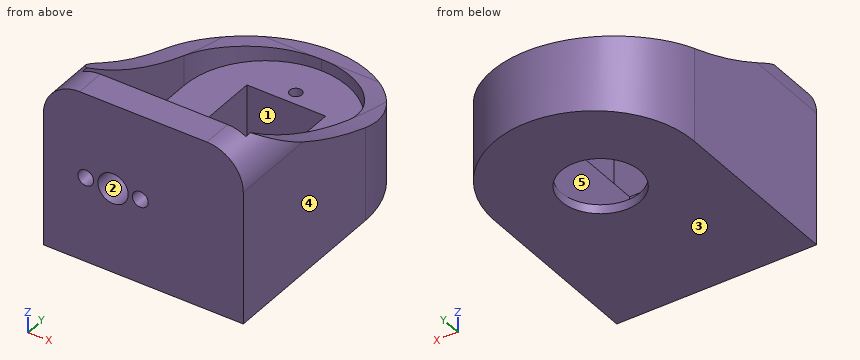
```python
from build123d import *

# Parameters (mm, degrees)
SKETCH1_W           = 33
SKETCH1_H           = 28
BOSS_EXTRUDE1_DEPTH = 46
SKETCH2_W           = 17.5
SKETCH2_H           = 41
CUT_EXTRUDE1_DEPTH  = 46
BOSS_EXTRUDE2_DEPTH = 3
BOSS_EXTRUDE3_DEPTH = 27
FILLET1_START       = -3.5
FILLET1_DEPTH       = 5.015993094
FILLET1_START_2     = -13.5
FILLET1_2_DEPTH     = 27
FILLET2_R           = 16.5
FILLET3_R           = 6
SKETCH5_W           = 13
SKETCH5_H           = 23
CUT_EXTRUDE4_DEPTH  = 9
SKETCH6_R           = 6.5
CUT_EXTRUDE5_DEPTH  = 9
SKETCH7_R           = 1
CUT_EXTRUDE6_DEPTH  = 8
SKETCH8_R           = 1.3
SKETCH8_R_2         = 2.5
CUT_EXTRUDE7_DEPTH  = 47.360004936


with BuildPart() as part:
    # Sketch1 → Boss-Extrude1 (new body)
    with BuildSketch(Plane(origin=(0, 0, 0), x_dir=(1, 0, 0), z_dir=(0, 1, 0))):
        Rectangle(SKETCH1_W, SKETCH1_H)
    extrude(amount=BOSS_EXTRUDE1_DEPTH)

    # Sketch2 → Cut-Extrude1 (cut)
    with BuildSketch(Plane(origin=(16.5, 0, 0), x_dir=(0, 0, -1), z_dir=(1, 0, 0))):
        with Locations((-5.25, 25.5)):
            Rectangle(SKETCH2_W, SKETCH2_H)
    extrude(amount=-CUT_EXTRUDE1_DEPTH, mode=Mode.SUBTRACT)

    # Sketch3 → Boss-Extrude2 (add)
    with BuildSketch(Plane(origin=(16.5, 0, 0), x_dir=(0, 0, -1), z_dir=(1, 0, 0))):
        with BuildLine():
            Line((3.5, 46), (2, 46))
            add(Edge.make_bspline(
                [(-14, 5), (-0.68227026, 23.158489921), (2, 46)],
                knots=[0, 0, 0, 1, 1, 1], degree=2))
            Line((-14, 5), (3.5, 5))
            Line((3.5, 5), (3.5, 46))
        make_face()
    boss_extrude2 = extrude(amount=-BOSS_EXTRUDE2_DEPTH)

    # Mirror1: Boss-Extrude2 across plane
    add(boss_extrude2.mirror(Plane(origin=(0, 0, 0), x_dir=(0, 0, 1), z_dir=(1, 0, 0))))

    # Sketch4 → Boss-Extrude3 (add)
    with BuildSketch(Plane.ZY.offset(-13.5)):
        with BuildLine():
            Line((-3.5, 46), (-3.5, 43))
            Line((-3.5, 43), (-1.598813094, 43))
            add(Edge.make_bspline(
                [(-1.598813094, 43), (-1.82265352, 44.489763885), (-2.000000005, 46.000000046)],
                knots=[0.933881948, 0.933881948, 0.933881948, 1, 1, 1], degree=2))
            Line((-2.000000005, 46.000000046), (-3.5, 46))
        make_face()
    extrude(amount=BOSS_EXTRUDE3_DEPTH)

    # Fillet1: read off the stored shape, not the designer's step
    # Fillet1 outline → Fillet1 (add)
    with BuildSketch(Plane.XY.offset(FILLET1_START)):
        with BuildLine():
            ThreePointArc((-13.5, 29.5), (-9.545941546, 39.045941546), (0, 43))
            Line((0, 43), (-13.5, 43))
            Line((-13.5, 43), (-13.5, 29.5))
        make_face()
        with BuildLine():
            ThreePointArc((0, 43), (9.545941546, 39.045941546), (13.5, 29.5))
            Line((13.5, 29.5), (13.5, 43))
            Line((13.5, 43), (0, 43))
        make_face()
    extrude(amount=FILLET1_DEPTH)

    # Fillet1 2 outline → Fillet1 2 (cut)
    with BuildSketch(Plane.YZ.offset(FILLET1_START_2)):
        with BuildLine():
            add(Edge.make_bspline(
                [(43, -1.598813094), (36.02565956, -0.550902514), (29.499999971, 1.515993003)],
                knots=[0.066118051, 0.066118051, 0.066118051, 0.375650194, 0.375650194, 0.375650194], degree=2))
            Line((43, -1.598813094), (43, 1.515993094))
            Line((43, 1.515993094), (29.499999971, 1.515993003))
        make_face()
    extrude(amount=FILLET1_2_DEPTH, mode=Mode.SUBTRACT)

    # Fillet2
    # the kernel refuses this fillet: 16.5 mm, written as the material it takes off along each edge
    with BuildSketch(Plane(origin=(16.5, 46, -55.25), x_dir=(0, -1, 0), z_dir=(0, 0, 1)), Plane(origin=(-16.5, 46, 39.25), x_dir=(0, -1, 0), z_dir=(0, 0, -1))) as fillet2_piece_1:
        with BuildLine():
            CenterArc((FILLET2_R, -FILLET2_R), FILLET2_R, 90, 90)
            Line((0, -FILLET2_R), (0, 0))
            Line((0, 0), (FILLET2_R, 0))
        make_face()
    extrude(amount=94.5, mode=Mode.SUBTRACT)

    # Fillet3
    # the kernel refuses this fillet: 6 mm, written as the material it takes off along each edge
    with BuildSketch(Plane(origin=(-16.5, -15, 14), x_dir=(1, 0, 0), z_dir=(0, 1, 0)), Plane(origin=(16.5, -15, 14), x_dir=(0, 0, -1), z_dir=(0, 1, 0))) as fillet3_piece_1:
        with BuildLine():
            CenterArc((FILLET3_R, FILLET3_R), FILLET3_R, 180, 90)
            Line((0, FILLET3_R), (0, 0))
            Line((0, 0), (FILLET3_R, 0))
        make_face()
    extrude(amount=35, mode=Mode.SUBTRACT)

    # Sketch5 → Cut-Extrude4 (cut)
    with BuildSketch(Plane.XY.offset(-3.5)):
        with Locations((0, 23)):
            Rectangle(SKETCH5_W, SKETCH5_H)
    extrude(amount=-CUT_EXTRUDE4_DEPTH, mode=Mode.SUBTRACT)

    # Sketch6 → Cut-Extrude5 (cut)
    with BuildSketch(Plane.XY.offset(-12.5)):
        with Locations((0, 28)):
            Circle(SKETCH6_R)
    extrude(amount=-CUT_EXTRUDE5_DEPTH, mode=Mode.SUBTRACT)

    # Sketch7 → Cut-Extrude6 (cut)
    with BuildSketch(Plane.XY.offset(-3.5)):
        with Locations((0, 36.8)):
            Circle(SKETCH7_R)
        with Locations((0, 9.2)):
            Circle(SKETCH7_R)
    extrude(amount=-CUT_EXTRUDE6_DEPTH, mode=Mode.SUBTRACT)

    # Sketch8 → Cut-Extrude7 (cut, through all)
    with BuildSketch(Plane(origin=(0, 5, 0), x_dir=(1, 0, 0), z_dir=(0, 1, 0))):
        with Locations(Location((-0.5, 0, 0), (0, 0, 270))):
            Circle(SKETCH8_R)
        with Locations(Location((-5, 0, 0), (0, 0, 270))):
            Circle(SKETCH8_R_2)
        with Locations(Location((-9.5, 0, 0), (0, 0, 270))):
            Circle(SKETCH8_R)
    extrude(amount=-CUT_EXTRUDE7_DEPTH, mode=Mode.SUBTRACT)


solid = part.part
```
Work out the finished part from the listing and answer in its coordinate system (mm). Face numbers are marked on the shaded views. A direction names the side the tool comes from. Coordinates: 2 decimals unless noted, no trailing zeros. Use CSV: the item, a comma, the result in double quotes.
1) Consider line 1 (X direction, y = 20, z = 1.25); line 2 (X direction, y = 2, z = 0); line 3 (X direction, y = 28, z = -13.45). Determine where each line is inside the solid, lowest interval first. Write a range as [from, to].
Worked out:
line 1,"x = [-16.5, -13.5], [13.5, 16.5]"
line 2,"x = [-16.5, -10.8], [-8.2, -7.5], [-2.5, -1.8], [0.8, 16.5]"
line 3,"x = [-16.5, -6.5], [6.5, 16.5]"
2) For the marked faces 4 and 5, determine the directions among +Z, -Z, +X, -X, +Y, -Y from which every point of the face is accessible in a straight line to the end or side of a thin tool.
Worked out:
face 4,"+Z, -Z, +X, +Y, -Y"
face 5,"+Z"
3) Section A-A on x = -5 is taken. Count the separate pieces of the cut face and the enclosed holes in it, plus the area to 3 significant figures.
Worked out:
separate pieces,"3"
enclosed holes,"0"
area,"324 mm^2"
4) Determine the mould class of the marked faces 1, 2 and 3 for opening direction Z: released by +Z, released by -Z, zero draft, split by the parting line, or undercut.
Worked out:
face 1,"zero draft"
face 2,"undercut"
face 3,"released by -Z"
5) Flat-ended cylindrical pins translate along their axes: pin 1 Ø5 at (x, z) = (-9, -9.5) entering from -Y; pin 2 Ø0.6 at (x, y) = (0, 36.5) entering from +Z; pin 3 Ø5 at (x, y) = (-4.5, 31.5) entering from +Z; pin 4 Ø2 at (y, z) = (11, 10) entering from +X. Find the tip coordinate at first contact, or state that the pin passes through.
Worked out:
pin 1,"stops at y = 0"
pin 2,"stops at z = -11.5"
pin 3,"stops at z = -3.5"
pin 4,"stops at x = 16.42"
